```python
from build123d import *

# Parameters (mm, degrees)
SKETCH1_R           = 125
SKETCH1_R_2         = 37.5
SKETCH1_R_3         = 25
BOSS_EXTRUDE1_DEPTH = 1050
SKETCH2_R           = 125
SKETCH2_R_2         = 25
BOSS_EXTRUDE2_DEPTH = 50
SHELL1_START        = -1090
SHELL1_DEPTH        = 1090
SHELL1_2_DEPTH      = 30


# Read off the part's stored shape, not the designer's step: Shell1
with BuildPart() as part:
    # Sketch1 → Boss-Extrude1 (new body)
    with BuildSketch(Plane(origin=(0, 0, 0), x_dir=(1, 0, 0), z_dir=(0, 1, 0))):
        with Locations(Location((0, 0, 0), (0, 0, 270))):
            Circle(SKETCH1_R)
        with Locations(Location((55, 55, 0), (0, 0, 270))):
            Circle(SKETCH1_R_2, mode=Mode.SUBTRACT)
        with Locations(Location((55, -55, 0), (0, 0, 270))):
            Circle(SKETCH1_R_2, mode=Mode.SUBTRACT)
        with Locations(Location((-55, -55, 0), (0, 0, 270))):
            Circle(SKETCH1_R_2, mode=Mode.SUBTRACT)
        with Locations(Location((-55, 55, 0), (0, 0, 270))):
            Circle(SKETCH1_R_2, mode=Mode.SUBTRACT)
        with Locations(Location((0, 0, 0), (0, 0, 270))):
            Circle(SKETCH1_R_3, mode=Mode.SUBTRACT)
    extrude(amount=-BOSS_EXTRUDE1_DEPTH)

    # Sketch2 → Boss-Extrude2 (add)
    with BuildSketch(Plane.XZ.offset(1050)):
        with Locations(Location((0, 0, 0), (0, 0, 90))):
            Circle(SKETCH2_R)
        with Locations(Location((0, 0, 0), (0, 0, 90))):
            Circle(SKETCH2_R_2, mode=Mode.SUBTRACT)
    extrude(amount=BOSS_EXTRUDE2_DEPTH)

    # Shell1 outline → Shell1 (cut)
    with BuildSketch(Plane(origin=(0, 0, 0), x_dir=(1, 0, 0), z_dir=(0, 1, 0)).offset(SHELL1_START)):
        with BuildLine():
            ThreePointArc((32.408845333, 13.216154667), (35, 0), (32.408845333, -13.216154667))
            ThreePointArc((32.408845333, -13.216154667), (78.149615303, -13.522954405), (102.422807797, -52.293101293))
            ThreePointArc((102.422807797, -52.293101293), (115, 0), (102.422807798, 52.293101293))
            ThreePointArc((102.422807798, 52.293101293), (78.149615303, 13.522954405), (32.408845333, 13.216154667))
        make_face()
        with BuildLine():
            ThreePointArc((-13.216154667, 32.408845333), (0, 35), (13.216154667, 32.408845333))
            ThreePointArc((13.216154667, 32.408845333), (13.522954405, 78.149615303), (52.293101293, 102.422807797))
            ThreePointArc((52.293101293, 102.422807797), (0, 115), (-52.293101293, 102.422807798))
            ThreePointArc((-52.293101293, 102.422807798), (-13.522954405, 78.149615303), (-13.216154667, 32.408845333))
        make_face()
        with BuildLine():
            ThreePointArc((52.293101293, -102.422807797), (13.522954405, -78.149615303), (13.216154667, -32.408845333))
            ThreePointArc((13.216154667, -32.408845333), (0, -35), (-13.216154667, -32.408845333))
            ThreePointArc((-13.216154667, -32.408845333), (-13.522954405, -78.149615303), (-52.293101293, -102.422807797))
            ThreePointArc((-52.293101293, -102.422807797), (0, -115), (52.293101293, -102.422807797))
        make_face()
        with BuildLine():
            ThreePointArc((-32.408845333, -13.216154667), (-35, 0), (-32.408845333, 13.216154667))
            ThreePointArc((-32.408845333, 13.216154667), (-78.149615303, 13.522954405), (-102.422807797, 52.293101293))
            ThreePointArc((-102.422807797, 52.293101293), (-115, 0), (-102.422807798, -52.293101293))
            ThreePointArc((-102.422807798, -52.293101293), (-78.149615303, -13.522954405), (-32.408845333, -13.216154667))
        make_face()
    extrude(amount=SHELL1_DEPTH, mode=Mode.SUBTRACT)

    # Shell1 2 outline → Shell1 2 (cut)
    with BuildSketch(Plane(origin=(0, 0, 0), x_dir=(1, 0, 0), z_dir=(0, 1, 0)).offset(SHELL1_START)):
        with BuildLine():
            ThreePointArc((13.216154667, 32.408845333), (24.748737342, 24.748737342), (32.408845333, 13.216154667))
            ThreePointArc((32.408845333, 13.216154667), (78.149615303, 13.522954405), (102.422807797, 52.293101293))
            ThreePointArc((102.422807797, 52.293101293), (81.317279836, 81.317279836), (52.293101293, 102.422807798))
            ThreePointArc((52.293101293, 102.422807798), (13.522954405, 78.149615303), (13.216154667, 32.408845333))
        make_face()
        with BuildLine():
            ThreePointArc((102.422807797, -52.293101293), (78.149615303, -13.522954405), (32.408845333, -13.216154667))
            ThreePointArc((32.408845333, -13.216154667), (24.748737342, -24.748737342), (13.216154667, -32.408845333))
            ThreePointArc((13.216154667, -32.408845333), (13.522954405, -78.149615303), (52.293101293, -102.422807797))
            ThreePointArc((52.293101293, -102.422807797), (81.317279836, -81.317279836), (102.422807797, -52.293101293))
        make_face()
        with BuildLine():
            ThreePointArc((-32.408845333, 13.216154667), (-24.748737342, 24.748737342), (-13.216154667, 32.408845333))
            ThreePointArc((-13.216154667, 32.408845333), (-13.522954405, 78.149615303), (-52.293101293, 102.422807797))
            ThreePointArc((-52.293101293, 102.422807797), (-81.317279836, 81.317279836), (-102.422807798, 52.293101293))
            ThreePointArc((-102.422807798, 52.293101293), (-78.149615303, 13.522954405), (-32.408845333, 13.216154667))
        make_face()
        with BuildLine():
            ThreePointArc((-52.293101293, -102.422807797), (-13.522954405, -78.149615303), (-13.216154667, -32.408845333))
            ThreePointArc((-13.216154667, -32.408845333), (-24.748737342, -24.748737342), (-32.408845333, -13.216154667))
            ThreePointArc((-32.408845333, -13.216154667), (-78.149615303, -13.522954405), (-102.422807797, -52.293101293))
            ThreePointArc((-102.422807797, -52.293101293), (-81.317279836, -81.317279836), (-52.293101293, -102.422807797))
        make_face()
    extrude(amount=SHELL1_2_DEPTH, mode=Mode.SUBTRACT)


solid = part.part
```
Work out the finished part from the listing and answer in its coordinate system (mm). A direction names the side the tool comes from. Give positions to 0.01 mm unless a question says otherwise; leave off trailing zeros. Loops run counter-clockwise (first coordinate to the right, second up) from the corner with the lowest first, then second, coordinate; pieces in that order, holes last. Notation, with made-up numbers: M 18,-31 L 44,-31 A30 ccw 44,-2 Z; hole C -6,37 d5. An arc over 180 degrees is marked long. One line per item, written item: value. Start each with the question number.
1. Find the intervals of material crossed by probe 1 along X at (y, z) = (-291, 55); probe 2 along X at (y, z) = (-626, -67.5); probe 3 along Y at (x, z) = (-38.5, 73), in increasing order.
2. Determine the mould class of faces 1 (the face through (66.26, -517.65, 90.77)), 2 (the face through (54, -1060, -56)), 3 (the face through (-56, -1050, -56)) for opening direction Y: released by +Y, released by -Y, zero draft, split by the parting line, or undercut.
3. Which of the six approach directions +Z, -Z, +X, -X, +Y, -Y give full straight-line access (tool end or side, diameter ignored) to faces 4 (the face through (-18, 0, -19)), 5 (the face through (54, -1050, 54)), 6 (the face through (-56, -1060, 54))?
4. Find section B-B (z = -66). Give the vertices of the cut face in (x, y), and give its area (3 significant figures).
5. Each of these flat-tipped pins is pushed along its axis until it touches: P1, Ø1, axis at y = -800.5, z = 96, coming from the -X side; P2, Ø25, axis at x = -69, z = -26, coming from the +Y side; P3, Ø22.5, axis at x = -60, z = -48, coming from the +Y side; P4, Ø10, axis at x = -31.5, y = -428, coming from the +Z side. Where does it stop, or does it pass through?
6. Find section A-A (y = -410.5). State how many separate pieces and enclosed holes the cut face has, and give its area (3 significant figures).
Reported:
1. probe 1: x = -112.25 to -92.5, -17.5 to -7.5, 7.5 to 17.5, 92.5 to 112.25
1. probe 2: x = -105.21 to -90.36, -19.64 to -9.17, 9.17 to 19.64, 90.36 to 105.21
1. probe 3: y = -1100 to -1090, -1060 to -1050
2. face 1: zero draft
2. face 2: undercut
2. face 3: released by +Y
3. face 4: +Z, -Z, +X, -X, +Y
3. face 5: +Y
3. face 6: none
4. outline: M -106.16,-1100 L 106.16,-1100 L 106.16,0 L 90.85,0 L 90.85,-1050 L 19.15,-1050 L 19.15,0 L 8.79,0 L 8.79,-1060 L 94.18,-1060 L 94.18,-1090 L -94.18,-1090 L -94.18,-1060 L -8.79,-1060 L -8.79,0 L -19.15,0 L -19.15,-1050 L -90.85,-1050 L -90.85,0 L -106.16,0 Z
4. area: 58,700 mm²
5. P1: stops at x = -80.65
5. P2: stops at y = 0
5. P3: stops at y = -1050
5. P4: stops at z = 122.16
6. separate pieces: 1
6. enclosed holes: 9
6. area: 17,700 mm²
